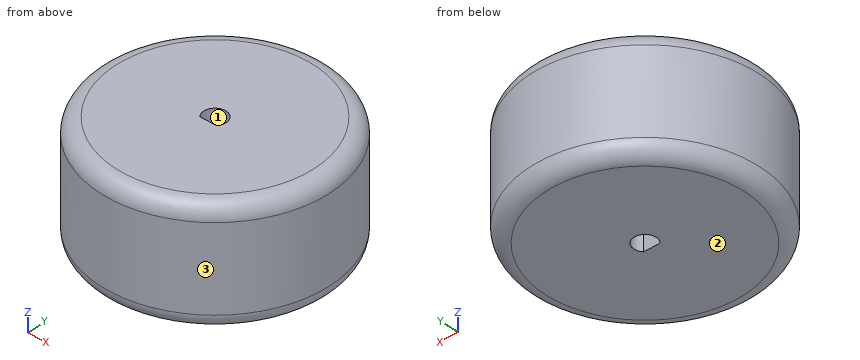
Autodesk Inventor part; units mm, degrees
ref_plane "YZ Plane" through (0, 0, 0) normal (1, 0, 0) x (0, 1, 0)
ref_plane "XZ Plane" through (0, 0, 0) normal (0, 1, 0) x (-1, 0, 0)
ref_plane "XY Plane" through (0, 0, 0) normal (0, 0, 1) x (1, 0, 0)
sketch "Sketch1" plane through (0, 0, 0) normal (0, 0, 1) x (1, 0, 0)
  circle A0 centre (0, 0) radius 15
  arc A1 (1.0844, -0.985) -> (-1.0844, -0.985) centre (0, 0) ccw
  line L0 (1.0844, -0.985) -> (-1.0844, -0.985)
  dimension "d0" = 30
  dimension "d1" = 2.93
  dimension "d2" = 2.45
extrude "Extrusion1" add sketch "Sketch1" along normal blind 15
fillet "Fillet1" radius 2 2 edges at (-15, 0, 15) (-15, 0, 0)
Verification items for the finished model (mm, model axes). Face numbers are marked on the shaded views. Give positions to 0.01 mm unless a question says otherwise; leave off trailing zeros. Loops run counter-clockwise (first coordinate to the right, second up) from the corner with the lowest first, then second, coordinate; pieces in that order, holes last.
1) Thickness scan on line 1 along Y through (x, z) = (0, 4.5) (3 decimals); line 2 along X through (y, z) = (-0.25, 1); line 3 along X through (y, z) = (8.25, 8.25). Record the ranges inside material, lowest first.
2) Sectioned sample at B-B, the plane y = 0. Enter the section's corners in (x, z), then the cut area to 3 significant figures.
3) Sectioned sample at D-D, the plane z = 13.5. Enter the section's corners in (x, y) (1 decimal).
4) Draft check along Y on the marked faces 1, 2 and 3. Enter one of: pulls with the +Y half, pulls with the -Y half, needs draft (parallel to the pull), parting line crosses it, or undercut.
5) Depth check by flat-ended pin: pin 1 Ø3 at (x, z) = (5, 11.5) entering from +Y; pin 2 Ø3 at (y, z) = (9, 5) entering from +X; pin 3 Ø4 at (x, z) = (8.5, 6.5) entering from -Y; pin 4 Ø1.8 at (x, y) = (0, 0) entering from +Z. Enter the tip coordinate at first touch or a pass-through.
6) Sectioned sample at C-C, the plane z = 7.75. Enter the section's corners in (x, y) (3 decimals).
7) Sectioned sample at A-A, the plane x = 0. Enter the section's corners in (y, z) (3 decimals), then the cut area to 3 significant figures.
Answers:
1. line 1: y = -15 to -0.985, 1.465 to 15
1. line 2: x = -14.73 to -1.44, 1.44 to 14.73
1. line 3: x = -12.53 to 12.53
2. outline: (-15, 2) arc R2 ccw to (-13, 0) - (-1.46, 0) - (-1.46, 15) - (-13, 15) arc R2 ccw to (-15, 13) - close; (1.46, 0) - (13, 0) arc R2 ccw to (15, 2) - (15, 13) arc R2 ccw to (13, 15) - (1.46, 15) - close
2. area: 403 mm2
3. outline: circle Ø29.9 at (0, 0); hole (-1.1, -1) - (1.1, -1) arc R1.5 ccw (long way) to start
4. face 1: undercut
4. face 2: needs draft
4. face 3: parting line crosses it
5. pin 1: stops at y = 14.59
5. pin 2: stops at x = 12.99
5. pin 3: stops at y = -13.52
5. pin 4: passes through
6. outline: circle Ø30 at (0, 0); hole (-1.084, -0.985) - (1.084, -0.985) arc R1.465 ccw (long way) to start
7. outline: (-15, 2) arc R2 ccw to (-13, 0) - (-0.985, 0) - (-0.985, 15) - (-13, 15) arc R2 ccw to (-15, 13) - close; (1.465, 0) - (13, 0) arc R2 ccw to (15, 2) - (15, 13) arc R2 ccw to (13, 15) - (1.465, 15) - close
7. area: 410 mm2
